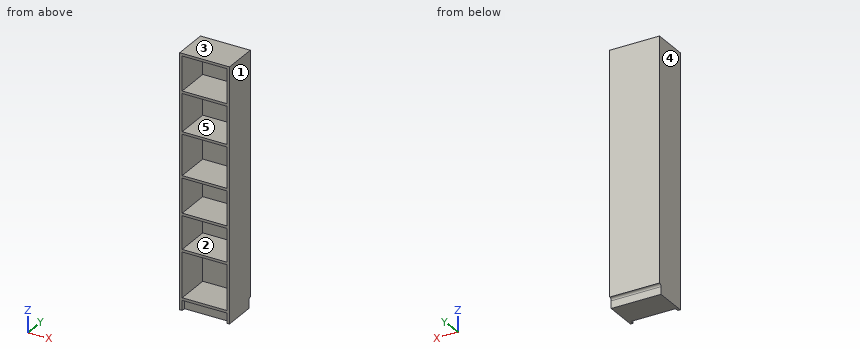
```python
from build123d import *

# Parameters (mm, degrees)
F0_W     = 400
F0_H     = 280
F1_DEPTH = 2020
F3_W     = 360
F3_H     = 275
F3_H_2   = 300
F3_H_3   = 325
F3_H_4   = 265
F3_H_5   = 360
F4_DEPTH = 277
F6_DEPTH = 400.001
F7_W     = 360
F7_H     = 80
F8_DEPTH = 30


with BuildPart() as f1:
    # F0 (on Top) → F1 (new body)
    with BuildSketch(Plane.XY):
        with Locations((0, -140)):
            Rectangle(F0_W, F0_H)
    extrude(amount=F1_DEPTH)

    # F3 (on face) → F4 (cut, through all)
    with BuildSketch(Plane.XZ.offset(280)):
        with Locations((0, 1862.5)):
            Rectangle(F3_W, F3_H)
        with Locations((0, 1555)):
            Rectangle(F3_W, F3_H_2)
        with Locations((0, 1222.5)):
            Rectangle(F3_W, F3_H_3)
        with Locations((0, 902.5)):
            Rectangle(F3_W, F3_H)
        with Locations((0, 612.5)):
            Rectangle(F3_W, F3_H_4)
        with Locations((0, 280)):
            Rectangle(F3_W, F3_H_5)
    extrude(amount=-F4_DEPTH, mode=Mode.SUBTRACT)

    # F5 (on face) → F6 (cut, through all)
    with BuildSketch(Plane(origin=(-200, 0, 0), x_dir=(0, -1, 0), z_dir=(-1, 0, 0))):
        with BuildLine():
            Line((0, 80), (0, 0))
            Line((0, 0), (20, 0))
            Line((20, 0), (20, 60))
            ThreePointArc((20, 60), (14.142136, 74.142136), (0, 80))
        make_face()
    extrude(amount=-F6_DEPTH, mode=Mode.SUBTRACT)

    # F7 (on face) → F8 (cut)
    with BuildSketch(Plane.XZ.offset(280)):
        with Locations((0, 40)):
            Rectangle(F7_W, F7_H)
    extrude(amount=-F8_DEPTH, mode=Mode.SUBTRACT)


solid = f1.part
```
CAD build for the part. Positions are in the model's coordinates, mm. Face numbers are marked on the shaded views. A direction names the side the tool comes from. Round coordinates to 2 decimals unless told otherwise and drop trailing zeros. Loops run counter-clockwise (first coordinate to the right, second up) from the corner with the lowest first, then second, coordinate; pieces in that order, holes last. Notation, with made-up numbers: (27.5, 88.25) - (50.5, 88.25) arc R30 cw to (50.5, 121.25) - close; hole circle Ø8 at (12, 12). An arc over 180 degrees is marked (long way). Return JSON: item names as keys, results as strings. Group by question number.
Q1. Band-saw the part on A-A on y = -201.5. Give the cut face in (x, z), plus the area to 3 significant figures.
Q2. Two-plate mould, pull along Z, no slides. Class the marked faces 1, 2 and 3: +Z half, -Z half, draft (parallel to the pull), parting line (faces both ways), or undercut.
Q3. Tool access for the marked faces 4 and 5: list every direction of +Z, -Z, +X, -X, +Y, -Y with a clear straight run to the whole face (end or side of a thin tool).
Q4. Band-saw the part on B-B on z = 155.5. Give the cut face in (x, y), plus the area to 3 significant figures.
Q5. Drill centre lines: line 1 along X through (y, z) = (-59, 538.5); line 2 along Y through (x, z) = (-44.5, 200.5). Where is each one in solid material? Low to high. Write a range as [from, to].
Solutions:
{
 "1": {"outline": "(-200, 0) - (200, 0) - (200, 2020) - (-200, 2020) - close; hole (-180, 100) - (180, 100) - (180, 460) - (-180, 460) - close; hole (-180, 480) - (180, 480) - (180, 745) - (-180, 745) - close; hole (-180, 765) - (180, 765) - (180, 1040) - (-180, 1040) - close; hole (-180, 1060) - (180, 1060) - (180, 1385) - (-180, 1385) - close; hole (-180, 1405) - (180, 1405) - (180, 1705) - (-180, 1705) - close; hole (-180, 1725) - (180, 1725) - (180, 2000) - (-180, 2000) - close", "area": "160,000 mm^2"},
 "2": {"face 1": "draft", "face 2": "undercut", "face 3": "+Z half"},
 "3": {"face 4": "+Z, -Z, -X, +Y, -Y", "face 5": "-Y"},
 "4": {"outline": "(-200, -280) - (-180, -280) - (-180, -3) - (180, -3) - (180, -280) - (200, -280) - (200, 0) - (-200, 0) - close", "area": "12,300 mm^2"},
 "5": {"line 1": "x = [-200, -180], [180, 200]", "line 2": "y = [-3, 0]"}
}
